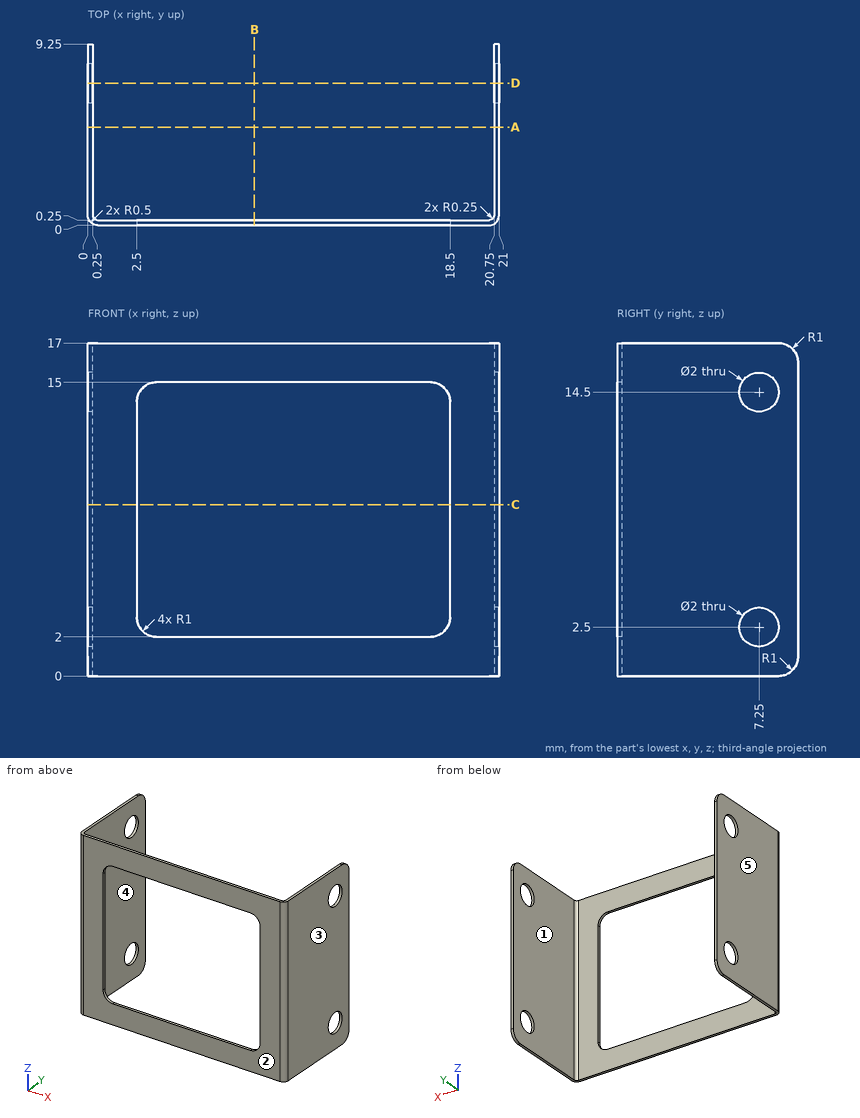
For this review, use the dimensioned drawing (mm, ordinates from the lowest corner) and the shaded views. A direction names the side the tool comes from. Round coordinates to 2 decimals unless told otherwise and drop trailing zeros. Write each loop counter-clockwise with the first axis right and the second up, starting at its lowest first coordinate (ties: lowest second). Pieces come first, ordered by that corner, then holes. Notation, with made-up numbers: (-28.75, 70.5) -> (9.25, 70.5) arc R29 cw to (9.25, 106.5) -> close; hole circle Ø10 at (88, -8.5). An arc over 180 degrees is marked (long way). One line per item, written item: value. Start each with the question number.
Q1. Tool access review of the marked faces 4 and 5: name each direction out of +Z, -Z, +X, -X, +Y, -Y from which nothing blocks a thin tool from reaching the whole face with its end or side.
Q2. To check wall thickness, follow probe 1 along Z at (x, y) = (20.9, 7.25); probe 2 along X at (y, z) = (2, 4); probe 3 along Y at (x, z) = (6.5, 1.25). State the ranges of each line that lie inside material, in increasing order.
Q3. Add section C-C (z = 8.75). Give the boundary of the cut face in (x, y), then the cut area to 3 significant figures.
Q4. The part is to be moulded in two halves that separate along X. For the marked faces 1, 2 and 3, say which applies: pulls with the +X half, pulls with the -X half, needs draft (parallel to the pull), parting line crosses it, or undercut.
Q5. Add section D-D (y = 7.25). Give the boundary of the cut face in (x, z).
Q6. Insertion check: P1, Ø8, axis at x = 4.5, z = 8.5, coming from the +Y side. The pin has a flat end and moves straight along its axis. Give the tip position at first contact, or say it passes through.
Q7. Add section B-B (x = 8.5). Give the boundary of the cut face in (y, z), then the cut area to 3 significant figures.
Q8. Add section A-A (y = 5). Give the boundary of the cut face in (x, z), then the cut area to 3 significant figures.
Response:
1. face 4: +Z, -Z, +Y
1. face 5: +Z, -Z, -X, +Y, -Y
2. probe 1: z = 0 to 1.5, 3.5 to 13.5, 15.5 to 17
2. probe 2: x = 0 to 0.25, 20.75 to 21
2. probe 3: y = 0 to 0.25
3. outline: (0, 0.5) arc R0.5 ccw to (0.5, 0) -> (2.5, 0) -> (2.5, 0.25) -> (0.5, 0.25) arc R0.25 cw to (0.25, 0.5) -> (0.25, 9.25) -> (0, 9.25) -> close; (18.5, 0) -> (20.5, 0) arc R0.5 ccw to (21, 0.5) -> (21, 9.25) -> (20.75, 9.25) -> (20.75, 0.5) arc R0.25 cw to (20.5, 0.25) -> (18.5, 0.25) -> close
3. area: 5.67 mm^2
4. face 1: undercut
4. face 2: needs draft
4. face 3: pulls with the +X half
5. outline: (0, 0) -> (0.25, 0) -> (0.25, 1.5) -> (0, 1.5) -> close; (0, 3.5) -> (0.25, 3.5) -> (0.25, 13.5) -> (0, 13.5) -> close; (0, 15.5) -> (0.25, 15.5) -> (0.25, 17) -> (0, 17) -> close; (20.75, 0) -> (21, 0) -> (21, 1.5) -> (20.75, 1.5) -> close; (20.75, 3.5) -> (21, 3.5) -> (21, 13.5) -> (20.75, 13.5) -> close; (20.75, 15.5) -> (21, 15.5) -> (21, 17) -> (20.75, 17) -> close
6. P1: stops at y = 0.25
7. outline: (0, 0) -> (0.25, 0) -> (0.25, 2) -> (0, 2) -> close; (0, 15) -> (0.25, 15) -> (0.25, 17) -> (0, 17) -> close
7. area: 1.00 mm^2
8. outline: (0, 0) -> (0.25, 0) -> (0.25, 17) -> (0, 17) -> close; (20.75, 0) -> (21, 0) -> (21, 17) -> (20.75, 17) -> close
8. area: 8.50 mm^2
